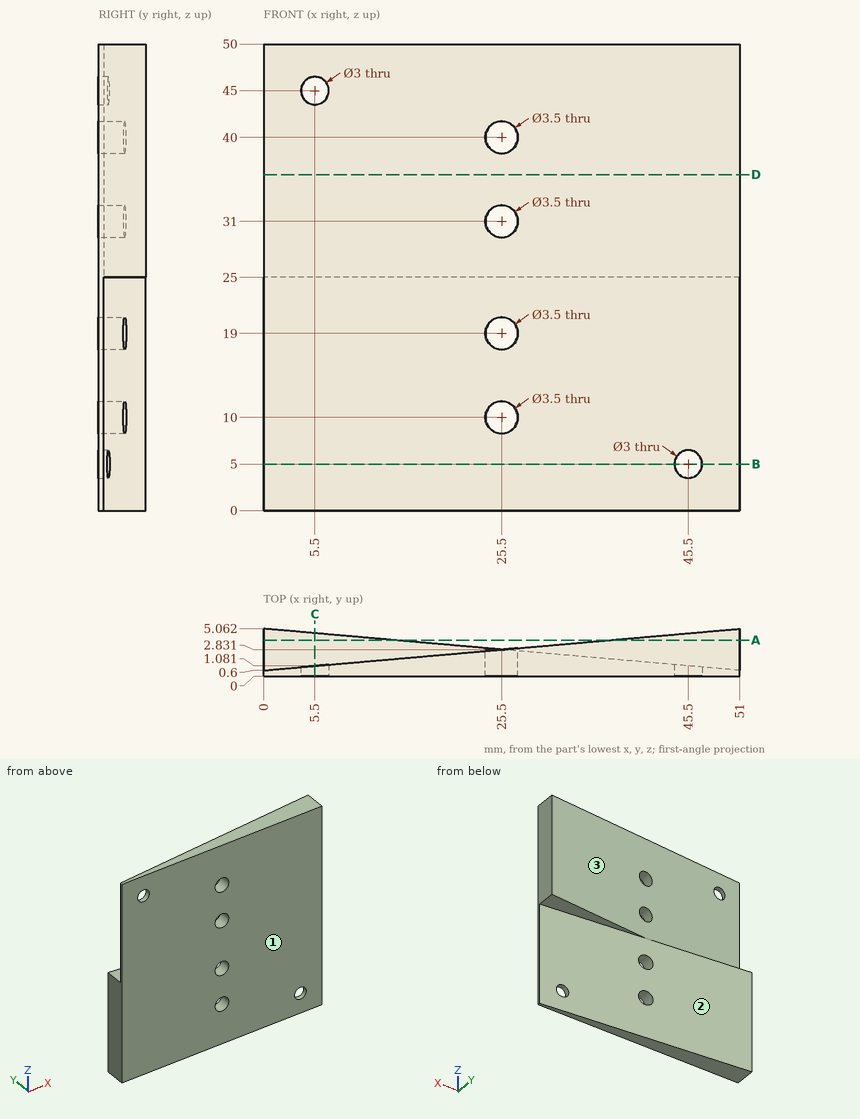
Verification items for this drawing (mm, ordinates from the low corner). A direction names the side the tool comes from. Give positions to 0.01 mm unless a question says otherwise; leave off trailing zeros. Loops run counter-clockwise (first coordinate to the right, second up) from the corner with the lowest first, then second, coordinate; pieces in that order, holes last. Notation, with made-up numbers: M 85.5,-9.5 L 90.5,-9.5 A19 ccw 90.5,15.5 Z; hole C 40.25,33 d7. An arc over 180 degrees is marked long. Answer as CSV lines item,"result".
Item 1: Cross-section at C-C on x = 5.5. Record the cut outline in (y, z), and give its area (3 significant figures).
Values:
outline,"M 0,0 L 4.58,0 L 4.58,25 L 1.08,25 L 1.08,43.5 L 0,43.5 Z; M 0,46.5 L 1.08,46.5 L 1.08,50 L 0,50 Z"
area,"138 mm²"
Item 2: Depth check by flat-ended pin: P1, Ø4.5, axis at x = 25.5, z = 40, coming from the -Y side; P2, Ø4, axis at x = 45.5, z = 5, coming from the +Y side; P3, Ø6, axis at x = 39.5, z = 13, coming from the +Y side; P4, Ø5.5, axis at x = 25.5, z = 31, coming from the +Y side. Enter the tip coordinate at first touch or a pass-through.
Values:
P1,"stops at y = 0"
P2,"stops at y = 1.26"
P3,"stops at y = 1.87"
P4,"stops at y = 3.07"
Item 3: Material ranges on line 1 (Z direction, x = 25.5, y = 2.1); line 2 (Z direction, x = 16, y = 2.05); line 3 (Z direction, x = 45.5, y = 0.7), recorded low to high.
Values:
line 1,"z = 0 to 8.25, 11.75 to 17.25, 20.75 to 29.25, 32.75 to 38.25, 41.75 to 50"
line 2,"z = 0 to 25"
line 3,"z = 0 to 3.5, 6.5 to 50"
Item 4: Cross-section at A-A on y = 3.85. Record the cut outline in (x, z), and give its area (3 significant figures).
Values:
outline,"M 0,0 L 13.85,0 L 13.85,25 L 0,25 Z; M 37.15,25 L 51,25 L 51,50 L 37.15,50 Z"
area,"693 mm²"
Item 5: Cross-section at B-B on z = 5. Record the cut outline in (x, y), and give its area (3 significant figures).
Values:
outline,"M 0,0 L 44,0 L 44,1.21 L 0,5.06 Z; M 47,0 L 51,0 L 51,0.6 L 47,0.95 Z"
area,"141 mm²"
Item 6: Cross-section at D-D on z = 36. Record the cut outline in (x, y).
Values:
outline,"M 0,0 L 51,0 L 51,5.06 L 0,0.6 Z"
Item 7: Access from +Z, -Z, +X, -X, +Y, -Y to the whole of each face (thin tool, end or side, straight path). Record for the marked faces 1, 2 and 3.
Values:
face 1,"+Z, -Z, +X, -X, -Y"
face 2,"-Z, +X, +Y"
face 3,"+Z, -X, +Y"
